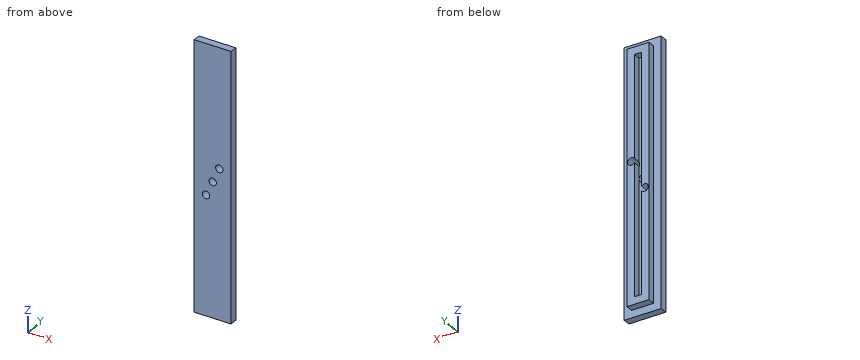
Autodesk Inventor part; units mm, degrees
ref_plane "YZ Plane" through (0, 0, 0) normal (1, 0, 0) x (0, 1, 0)
ref_plane "XZ Plane" through (0, 0, 0) normal (0, 1, 0) x (-1, 0, 0)
ref_plane "XY Plane" through (0, 0, 0) normal (0, 0, 1) x (1, 0, 0)
sketch "Sketch1" plane through (0, 0, 0) normal (0, 1, 0) x (-1, 0, 0)
  line L0 (0, 0) -> (0, -114.3)
  line L1 (0, -114.3) -> (-15.875, -114.3)
  line L2 (-15.875, -114.3) -> (-15.875, 0)
  line L3 (-15.875, 0) -> (0, 0)
  dimension "d0" = 114.3
  dimension "d1" = 15.875
extrude "Extrusion1" add sketch "Sketch1" along normal blind 3.175
sketch "Sketch2" plane through (0, 3.175, 0) normal (0, 1, 0) x (1, 0, 0)
  line L0 (0, 0) -> (3.175, 0)
  line L1 (0, 0) -> (15.875, 0)
  line L2 (3.175, 0) -> (3.175, 3.175)
  line L3 (3.175, 3.175) -> (6.35, 3.175)
  line L4 (6.35, 3.175) -> (6.35, 111.125)
  line L5 (6.35, 111.125) -> (3.175, 111.125)
  line L6 (3.175, 111.125) -> (3.175, 3.175)
  line L7 (15.875, 0) -> (15.875, 114.3)
  dimension "d4" = 3.175
  dimension "d5" = 3.175
  dimension "d6" = 3.175
  dimension "d7" = 107.95
extrude "Extrusion2" add sketch "Sketch2" along normal blind 3.175
sketch "Sketch3" plane through (0, 3.175, 0) normal (0, 1, 0) x (1, 0, 0)
  line L0 (15.875, 0) -> (15.875, 114.3)
  line L1 (15.875, 0) -> (12.7, 0)
  line L2 (0, 0) -> (15.875, 0)
  line L3 (12.7, 0) -> (12.7, 3.175)
  line L4 (12.7, 3.175) -> (9.525, 3.175)
  line L5 (9.525, 3.175) -> (9.525, 111.125)
  line L6 (9.525, 111.125) -> (12.7, 111.125)
  line L7 (12.7, 111.125) -> (12.7, 3.175)
  dimension "d10" = 3.175
  dimension "d11" = 3.175
  dimension "d12" = 3.175
  dimension "d13" = 107.95
extrude "Extrusion3" add sketch "Sketch3" along normal blind 3.175
sketch "Sketch4" plane through (0, 3.175, 0) normal (0, 1, 0) x (1, 0, 0)
  line L0 (6.35, 3.175) -> (3.175, 3.175)
  line L1 (6.35, 3.175) -> (9.525, 3.175)
  line L2 (9.525, 3.175) -> (9.525, 6.35)
  line L3 (9.525, 6.35) -> (6.35, 6.35)
  line L4 (6.35, 6.35) -> (6.35, 3.175)
  point P0 (0, 0)
  dimension "d16" = 3.175
  dimension "d17" = 3.175
extrude "Extrusion4" add sketch "Sketch4" along normal blind 3.175
sketch "Sketch5" plane through (0, 3.175, 0) normal (0, 1, 0) x (1, 0, 0)
  line L0 (6.35, 6.35) -> (6.35, 111.125)
  line L1 (6.35, 111.125) -> (9.525, 111.125)
  line L2 (9.525, 111.125) -> (9.525, 107.95)
  line L3 (9.525, 107.95) -> (6.35, 107.95)
  line L4 (6.35, 107.95) -> (6.35, 111.125)
  point P0 (0, 0)
  dimension "d20" = 3.175
  dimension "d21" = 3.175
extrude "Extrusion5" add sketch "Sketch5" along normal blind 3.175
sketch "Sketch6" plane through (0, 3.175, 0) normal (0, 1, 0) x (1, 0, 0)
  line L0 (0, 0) -> (7.9375, 0)
  line L1 (0, 0) -> (15.875, 0)
  line L2 (7.9375, 0) -> (7.9375, 57.15)
  dimension "d24" = 7.9375
  dimension "d25" = 57.15
hole "Hole1" at (7.9375, 3.175, -57.15) direction (0, -1, 0) diameter 3.175 end through all
sketch "Sketch10" plane through (0, 0, 0) normal (0, -1, 0) x (1, 0, 0)
  line L0 (15.875, 0) -> (15.875, -114.3)
  line L1 (15.875, 0) -> (15.875, -50.8)
  line L2 (15.875, -50.8) -> (10.795, -50.8)
  point P0 (0, 0)
  dimension "d46" = 50.8
  dimension "d47" = 5.08
hole "Hole3" at (10.795, 0, -50.8) direction (0, 1, 0) diameter 3.175 end through all
sketch "Sketch11" plane through (0, 0, 0) normal (0, -1, 0) x (1, 0, 0)
  line L0 (0, 0) -> (0, -63.5)
  line L1 (0, -114.3) -> (0, 0)
  line L2 (0, -63.5) -> (5.08, -63.5)
  dimension "d55" = 63.5
  dimension "d56" = 5.08
hole "Hole4" at (5.08, 0, -63.5) direction (0, 1, 0) diameter 3.175 end through all
properties part number "single_cell_top_case"
Geometry check sheet. Reference: the model listing, model coordinates, mm. Round coordinates to 2 decimals unless told otherwise and drop trailing zeros. Loops run counter-clockwise (first coordinate to the right, second up) from the corner with the lowest first, then second, coordinate; pieces in that order, holes last. Notation, with made-up numbers: (84.25, 1.5) - (133.25, 1.5) arc R13 ccw to (133.25, 19.5) - close; hole circle Ø8 at (-6, 27). An arc over 180 degrees is marked (long way). Use a Markdown table: item, result.
Q1. Cross-section at C-C on x = 1.25. Record the cut outline in (y, z) (3 decimals).
Solutions:
| item | result |
|---|---|
| outline | (0, -114.3) - (3.175, -114.3) - (3.175, 0) - (0, 0) - close |
Q2. Go/stop test with flat-tipped pins: P1, Ø3.5, axis at x = 9.5, y = 5, coming from the +Z side (3 decimals); P2, Ø4, axis at x = 10.795, z = -50.8, coming from the -Y side; P3, Ø1, axis at x = 7.5, y = 4, coming from the -Z side (3 decimals); P4, Ø2, axis at y = 5, z = -90, coming from the -X side (3 decimals). Record where each tip stops, or that it passes through.
Solutions:
| item | result |
|---|---|
| P1 | stops at z = -3.175 |
| P2 | stops at y = 0 |
| P3 | stops at z = -111.125 |
| P4 | stops at x = 3.175 |
Q3. Material ranges on line 1 (Z direction, x = 5, y = 3); line 2 (X direction, y = 1.35, z = -57.15) (3 decimals); line 3 (X direction, y = 6, z = -67) (3 decimals), recorded low to high.
Solutions:
| item | result |
|---|---|
| line 1 | z = -114.3 to -65.09, -61.91 to 0 |
| line 2 | x = 0 to 6.35, 9.525 to 15.875 |
| line 3 | x = 3.175 to 6.35, 9.525 to 12.7 |
